The listing builds one solid part. Answer for the finished solid, in the listing's coordinates (mm). Give positions to 0.01 mm unless a question says otherwise; leave off trailing zeros. Write each loop counter-clockwise with the first axis right and the second up, starting at its lowest first coordinate (ties: lowest second). Pieces come first, ordered by that corner, then holes. Notation, with made-up numbers: (-38.75, 35.5) -> (8.25, 35.5) arc R29 ccw to (8.25, 56.5) -> close; hole circle Ø2 at (8.5, 59.25). An arc over 180 degrees is marked (long way). Write each question's results on one line, items separated by ' | '. Start each with the question number.
Autodesk Inventor part; units mm, degrees
ref_plane "YZ Plane" through (0, 0, 0) normal (1, 0, 0) x (0, 1, 0)
ref_plane "XZ Plane" through (0, 0, 0) normal (0, 1, 0) x (-1, 0, 0)
ref_plane "XY Plane" through (0, 0, 0) normal (0, 0, 1) x (1, 0, 0)
sketch "Sketch1" plane through (0, 0, 0) normal (0, 1, 0) x (-1, 0, 0)
  line L0 (101.6, 38.1) -> (-101.6, 38.1) construction
  line L1 (-101.6, 38.1) -> (-101.6, -38.1) construction
  line L2 (-101.6, -38.1) -> (101.6, -38.1) construction
  line L3 (101.6, -38.1) -> (101.6, 38.1) construction
  line L4 (101.6, 38.1) -> (-101.6, -38.1) construction
  line L5 (-101.6, 38.1) -> (101.6, -38.1) construction
  line L6 (-28.575, 66.675) -> (28.575, 66.675) construction
  line L7 (28.575, 66.675) -> (28.575, 9.525)
  line L8 (28.575, 9.525) -> (-28.575, 9.525)
  line L9 (-28.575, 9.525) -> (-28.575, 66.675)
  line L10 (-28.575, 66.675) -> (28.575, 9.525) construction
  line L11 (28.575, 66.675) -> (-28.575, 9.525) construction
  circle A0 centre (-38.1, 50.8) radius 3.175
  line L12 (0, 38.1) -> (0, -38.1) construction
  circle A1 centre (-38.1, 50.8) radius 9.525
  line L13 (-38.1, 60.325) -> (-28.575, 60.325)
  circle A2 centre (38.1, 50.8) radius 3.175
  circle A3 centre (38.1, 50.8) radius 9.525
  line L14 (38.1, 60.325) -> (28.575, 60.325)
  circle A4 centre (-76.2, -38.1) radius 1.7526
  circle A5 centre (-95.25, 3.175) radius 1.7526
  circle A6 centre (76.2, -38.1) radius 1.7526
  circle A7 centre (95.25, 3.175) radius 1.7526
  line L15 (-101.6, -38.1) -> (-101.6, 6.35)
  line L16 (-101.6, 6.35) -> (-44.4797, 57.8728)
  line L17 (101.6, -38.1) -> (101.6, 6.35)
  line L18 (101.6, 6.35) -> (44.4797, 57.8728)
  line L19 (-42.6417, 42.4275) -> (-87.975, 1.5367)
  line L20 (-87.975, 1.5367) -> (-87.975, -38.1)
  line L21 (87.975, -38.1) -> (87.975, 1.5367)
  line L22 (87.975, 1.5367) -> (42.6417, 42.4275)
  line L23 (0, -38.1) -> (-95.25, -38.1) construction
  line L24 (0, -38.1) -> (95.25, -38.1) construction
  circle A8 centre (-60.325, 35.0287) radius 1.7526
  circle A9 centre (-33.3375, 31.75) radius 1.7526
  line L25 (-38.1, 0) -> (-38.1, 41.275)
  line L26 (-38.1, 0) -> (0, 0) construction
  circle A10 centre (60.325, 35.0287) radius 1.7526
  circle A11 centre (33.3375, 31.75) radius 1.7526
  line L27 (38.1, 0) -> (38.1, 41.275)
  line L28 (38.1, 0) -> (0, 0) construction
  line L29 (-87.975, 0) -> (-65.115, 0)
  line L30 (-65.115, 0) -> (-65.115, -31.75)
  line L31 (-65.115, -31.75) -> (-87.975, -31.75)
  line L32 (-101.6, -38.1) -> (101.6, -38.1) construction
  line L33 (101.6, -38.1) -> (101.6, 19.05)
  line L34 (101.6, 19.05) -> (-101.6, 19.05) construction
  line L35 (-101.6, 19.05) -> (-101.6, -38.1)
  line L36 (-101.6, 19.05) -> (-87.5203, 19.05) construction
  line L37 (87.5203, 19.05) -> (101.6, 19.05) construction
  circle A12 centre (-38.1, 0) radius 3.175 construction
  circle A13 centre (-38.1, 0) radius 6.35 construction
  circle A14 centre (38.1, 0) radius 3.175 construction
  circle A15 centre (38.1, 0) radius 6.35 construction
  circle A16 centre (28.575, 9.525) radius 1.7526
  circle A17 centre (28.575, 9.525) radius 4.7625
  arc A18 (17.0773, 9.525) -> (28.575, 21.0227) centre (17.0773, 21.0227) ccw
  circle A19 centre (-28.575, 9.525) radius 1.7526
  circle A20 centre (-28.575, 9.525) radius 4.7625
  arc A21 (-28.575, 21.0227) -> (-17.0773, 9.525) centre (-17.0773, 21.0227) ccw
  arc A22 (31.4325, 5.715) -> (38.1, 19.05) centre (21.4312, 19.05) ccw
  arc A23 (-38.1, 19.05) -> (-31.4325, 5.715) centre (-21.4312, 19.05) ccw
  line L38 (-61.94, -38.1) -> (-61.94, 25.0204)
  line L39 (87.975, 0) -> (65.115, 0)
  line L40 (65.115, 0) -> (65.115, -31.75)
  line L41 (65.115, -31.75) -> (87.975, -31.75)
  line L42 (61.94, -38.1) -> (61.94, 25.0204)
  line L43 (-28.575, 4.7625) -> (28.575, 4.7625)
  line L44 (101.6, -31.75) -> (-101.6, -31.75)
  line L45 (-101.6, -31.75) -> (-101.6, -44.45) construction
  line L46 (-101.6, -44.45) -> (101.6, -44.45)
  line L47 (101.6, -44.45) -> (101.6, -31.75) construction
  circle A24 centre (0, -38.1) radius 1.7526
  circle A25 centre (38.1, -38.1) radius 1.7526
  circle A26 centre (-38.1, -38.1) radius 1.7526
  line L48 (101.6, -38.1) -> (76.2, -44.45)
  line L49 (-101.6, -38.1) -> (-76.2, -44.45)
  line L50 (76.2, -38.1) -> (76.2, -44.45) construction
  line L51 (-76.2, -38.1) -> (-76.2, -44.45) construction
  line L52 (59.1924, 41.2769) -> (32.488, 36.4361)
  circle A27 centre (60.325, 35.0287) radius 6.35
  circle A28 centre (33.3375, 31.75) radius 4.7625
  line L53 (-59.1924, 41.2769) -> (-32.488, 36.4361)
  circle A29 centre (-60.325, 35.0287) radius 6.35
  circle A30 centre (-33.3375, 31.75) radius 4.7625
  line L54 (-87.975, 0) -> (-65.115, 0)
  line L55 (-65.115, 0) -> (-65.115, -3.175)
  line L56 (-65.115, -3.175) -> (-87.975, -3.175)
  line L57 (-87.975, -3.175) -> (-87.975, 0)
  line L58 (-65.115, -15.875) -> (-87.975, -15.875) construction
  line L59 (-65.115, -28.575) -> (-87.975, -28.575)
  line L60 (-84.8, -38.1) -> (-84.8, 0.1248)
  line L61 (65.115, -3.175) -> (87.975, -3.175)
  line L62 (65.115, -15.875) -> (87.975, -15.875) construction
  line L63 (65.115, -28.575) -> (87.975, -28.575)
  line L64 (84.8, -38.1) -> (84.8, 0.1248)
  point P0 (28.575, 38.1)
  point P1 (-28.575, 38.1)
  point P2 (28.575, 60.325)
  point P3 (44.4797, 57.8728)
  point P4 (101.6, -15.875)
  point P5 (38.1, 41.275)
  point P6 (-87.975, -31.75)
  point P7 (-101.6, 6.35)
  point P8 (101.6, 6.35)
  point P9 (31.75, 0)
  point P10 (38.1, 6.35)
  point P11 (-38.1, 6.35)
  point P12 (-31.75, 0)
  point P13 (87.975, 0)
  point P14 (61.94, 25.0204)
  point P15 (-17.0773, 9.525)
  point P16 (-28.575, 21.0227)
  point P17 (-38.1, 19.05)
  point P18 (-31.4325, 5.715)
  point P19 (-21.8502, 0)
  point P20 (21.8502, 0)
  point P21 (-25.2074, 12.8926)
  point P22 (-28.575, 14.2875)
  point P23 (-23.8125, 9.525)
  point P24 (-28.575, 50.8)
  point P25 (25.2074, 12.8926)
  point P26 (28.575, 14.2875)
  point P27 (23.8125, 9.525)
  point P28 (28.575, 50.8)
  point P29 (26.8224, 9.525)
  point P30 (28.575, 11.2776)
  point P31 (61.94, -31.75)
  point P32 (-61.94, -31.75)
  point P33 (-28.575, 31.75)
  point P34 (-64.5781, 39.7439)
  point P35 (64.5781, 39.7439)
  point P36 (28.575, 31.75)
  point P37 (-84.8, -3.175)
  point P38 (-84.8, -28.575)
  point P39 (84.8, -3.175)
  point P40 (84.8, -28.575)
  point P41 (-101.6, -31.75)
  point P42 (-56.0719, 30.3135)
  point P43 (56.0719, 30.3135)
  point P44 (46.4735, 38.9713)
  point P45 (-46.4735, 38.9713)
  point P46 (-28.575, 11.2776)
  point P47 (-26.8224, 9.525)
  dimension "d0" = 203.2
  dimension "d1" = 76.2
  dimension "d4" = 57.15
  dimension "d6" = 6.35
  dimension "d7" = 38.1
  dimension "d8" = 19.05
  dimension "d10" = 3.5052
  dimension "d11" = 3.5052
  dimension "d12" = 0
  dimension "d14" = 25.4
  dimension "d15" = 6.35
  dimension "d20" = 50.8
  dimension "d21" = 41.275
  dimension "d22" = 44.45
  dimension "d24" = 12.7
  dimension "d25" = 13.625
  dimension "d26" = 12.7
  dimension "d27" = 13.625
  dimension "d31" = 3.5052
  dimension "d32" = 3.5052
  dimension "d33" = 6.35
  dimension "d34" = 31.75
  dimension "d35" = 4.7625
  dimension "d36" = 22.225
  dimension "d37" = 9.525
  dimension "d39" = 31.75
  dimension "d40" = 6.35
  dimension "d42" = 57.15
  dimension "d43" = 6.35
  dimension "d44" = 9.525
  dimension "d45" = 9.525
  dimension "d46" = 12.7
  dimension "d104" = 3.5052
  dimension "d105" = 9.525
  dimension "d106" = 3.175
  dimension "d107" = 22.86
  dimension "d123" = 88.9
  dimension "d124" = 12.7
  dimension "d125" = 3.5052
  dimension "d126" = 3.5052
  dimension "d127" = 38.1
  dimension "d128" = 28.575
  dimension "d129" = 3.175
  dimension "d130" = 3.175
extrude "Extrusion1" add sketch "Sketch1" along normal blind 3.175 contours A28 L27 A22 A17 L7 | A28 | L7 A17 A18 | L52 L27 A28 | L27 L52 L22 L42 L44 L38 L19 L53 L25 A23 A20 L43 A17 A22 | L18 L17 L44 L21 L22 A27 | A27 | A17 L8 A16 L7 | L7 A16 L8 A17 | A17 L8 A18 | L52 A27 L22 | A17 L43 A20 L8 | L17 L48 L46 L49 L15 L44 L31 L41 | L8 A20 A21 | L22 L21 L39 L40 L44 L42 | L41 L64 L63 L21 | A20 L9 A19 L8 | L8 A19 L9 A20 | A20 L9 A21 | L63 L64 L61 L21 | L41 L40 L63 L64 | A23 L25 A30 L9 A20 | L21 L61 L64 L39 | L44 L30 L29 L20 L19 L38 | A30 | L64 L61 L40 L39 | L19 L20 L44 L15 L16 A29 | L31 L60 L59 L30 | L25 L53 A30 | A29 L53 L19 | A29 | L31 L20 L59 L60 | L29 L60 L56 L20 | L56 L60 L29 L30 | L59 L20 L56 L60
fillet "Fillet1" radius 6.35 14 edges at (101.6, 1.5875, -38.1) (101.6, 1.5875, 6.35) (-101.6, 1.5875, 6.35) (76.2, 1.5875, -44.45) (-76.2, 1.5875, -44.45) (-101.6, 1.5875, -38.1) (-65.115, 1.5875, -3.175) (-65.115, 1.5875, -28.575) (-84.8, 1.5875, -3.175) (-84.8, 1.5875, -28.575) (84.8, 1.5875, -3.175) (65.115, 1.5875, -3.175) (84.8, 1.5875, -28.575) (65.115, 1.5875, -28.575)
equation "\"d35\" = 0.5 * d37"
properties part number "Chassis" material "UHMW, Black"
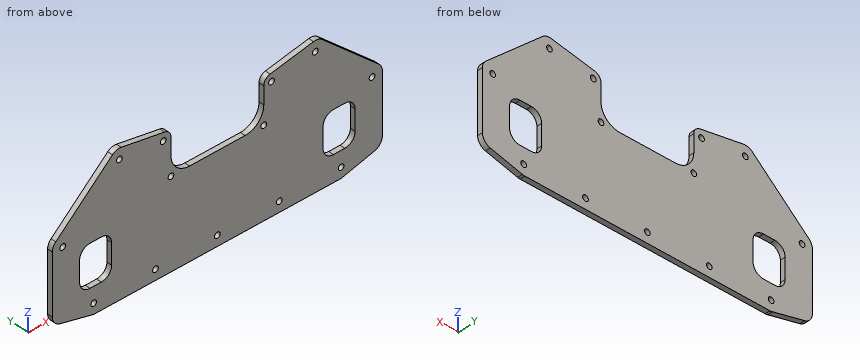
1. Section B-B (z = 15.5) is taken. Write down the section's boundary in (x, y) (3 decimals).
2. Section A-A (x = 82.5) is taken. Write down the section's boundary in (y, z) (3 decimals).
3. Section D-D (x = -88) is taken. Write down the section's boundary in (y, z) (3 decimals), then the cut area to 3 significant figures.
4. Consider probe 1 along X at (y, z) = (0.65, -19) (3 decimals); probe 2 along X at (y, z) = (2.2, 31.5) (3 decimals); probe 3 along X at (y, z) = (2.45, -6). Determine where each line is inside the solid, lowest interval first. Write a range as [from, to].
5. Section C-C (y = 1.5) is taken. Give the number of separate pieces and of enclosed holes in the cut face, then the cut area to 3 significant figures.
6. Each of these flat-tipped pins is pushed along its axis until it touches: pin 1 Ø5.5 at (x, z) = (95.25, 3.175) entering from -Y; pin 2 Ø1 at (x, y) = (-76.5, 2) entering from +Z; pin 3 Ø1 at (x, y) = (75, 1.5) entering from +Z; pin 4 Ø3 at (x, z) = (-28.575, 9.525) entering from +Y. Where does it stop, or does it pass through?
Results:
1) outline: (-91.456, 0) -> (-27.162, 0) -> (-27.162, 3.175) -> (-91.456, 3.175) -> close; (27.162, 0) -> (91.456, 0) -> (91.456, 3.175) -> (27.162, 3.175) -> close
2) outline: (0, -42.875) -> (3.175, -42.875) -> (3.175, -27.116) -> (0, -27.116) -> close; (0, -4.634) -> (3.175, -4.634) -> (3.175, 23.578) -> (0, 23.578) -> close
3) outline: (0, -41.5) -> (3.175, -41.5) -> (3.175, 18.617) -> (0, 18.617) -> close | area: 191 mm²
4) probe 1: x = [-101.6, -84.8], [-65.115, 65.115], [84.8, 101.6] | probe 2: x = [-73.718, -35.072], [-31.603, -28.575], [28.575, 31.603], [35.072, 73.718] | probe 3: x = [-101.6, -83.73], [-66.18, 66.18], [83.73, 101.6]
5) separate pieces: 1 | enclosed holes: 15 | area: 12,900 mm²
6) pin 1: stops at y = 0 | pin 2: stops at z = 29.44 | pin 3: stops at z = 30.79 | pin 4: passes through
